Design review of the part built by this model. Coordinates are the model's own, in mm. A direction names the side the tool comes from. Coordinates: 2 decimals unless noted, no trailing zeros. Write each loop counter-clockwise with the first axis right and the second up, starting at its lowest first coordinate (ties: lowest second). Pieces come first, ordered by that corner, then holes. Notation, with made-up numbers: M 73.25,53 L 116.25,53 A10 ccw 116.25,69 Z; hole C 55.5,63 d4. An arc over 180 degrees is marked long. Return JSON: item names as keys, results as strings. Group by question number.
Autodesk Fusion 360 part; units mm, degrees
sketch "Sketch1" plane through (0, 0, 0) normal (0, 0, 1) x (1, 0, 0)
  line L0 (0, 0) -> (324.3, 0)
  line L1 (324.3, 0) -> (324.3, 429.3)
  line L2 (324.3, 429.3) -> (0, 429.3)
  line L3 (0, 429.3) -> (0, 0)
  dimension "d7" = 324.3
  dimension "d8" = 429.3
extrude "Extrude1" add sketch "Sketch1" along normal blind 55
fillet "Fillet1" radius 8 4 edges at (324.3, 0, 27.5) (324.3, 429.3, 27.5) (0, 429.3, 27.5) (0, 0, 27.5)
shell "Shell1" thickness 5 removed faces 1 at (216.2, 283.5333, 55)
ref_plane "WorkPlane1" through (162.15, 214.65, 50) normal (0, 0, 1) x (1, 0, 0)
sketch "Sketch2" plane through (0, 0, 50) normal (0, 0, 1) x (1, 0, 0)
  line L0 (10, 427.3) -> (314.3, 427.3)
  line L1 (322.3, 419.3) -> (322.3, 10)
  line L2 (314.3, 2) -> (10, 2)
  line L3 (2, 10) -> (2, 419.3)
  arc A0 (8, 424.3) -> (5, 421.3) centre (8, 421.3) ccw
  line L4 (8, 424.3) -> (316.3, 424.3)
  arc A1 (319.3, 421.3) -> (316.3, 424.3) centre (316.3, 421.3) ccw
  line L5 (319.3, 421.3) -> (319.3, 8)
  arc A2 (316.3, 5) -> (319.3, 8) centre (316.3, 8) ccw
  line L6 (316.3, 5) -> (8, 5)
  arc A3 (5, 8) -> (8, 5) centre (8, 8) ccw
  line L7 (5, 8) -> (5, 421.3)
  arc A4 (0, 8) -> (8, 0) centre (8, 8) ccw
  line L8 (8, 0) -> (316.3, 0)
  arc A5 (316.3, 0) -> (324.3, 8) centre (316.3, 8) ccw
  line L9 (324.3, 8) -> (324.3, 421.3)
  arc A6 (324.3, 421.3) -> (316.3, 429.3) centre (316.3, 421.3) ccw
  line L10 (316.3, 429.3) -> (8, 429.3)
  arc A7 (8, 429.3) -> (0, 421.3) centre (8, 421.3) ccw
  line L11 (0, 421.3) -> (0, 8)
  arc A8 (2, 10) -> (10, 2) centre (10, 10) ccw
  arc A9 (10, 427.3) -> (2, 419.3) centre (10, 419.3) ccw
  arc A10 (322.3, 419.3) -> (314.3, 427.3) centre (314.3, 419.3) ccw
  arc A11 (314.3, 2) -> (322.3, 10) centre (314.3, 10) ccw
  dimension "d19" = 2
  dimension "d20" = 2
  dimension "d21" = 2
  dimension "d22" = 2
  dimension "d23" = 8
extrude "Extrude2" cut sketch "Sketch2" along normal through all contours L0 L1 L2 L3 A8 A9 A10 A11
fillet "Fillet2" radius 8 1 faces at (216.2, 283.5333, 0)
equation "tray_depth = panel_depth + 2 * ( wall_thickness - lip_thickness ) + printer_tolerance"
equation "tray_width = panel_width + 2 * ( wall_thickness - lip_thickness ) + printer_tolerance"
equation "wall_height = 55 mm"
equation "wall_thickness = 2 mm + lip_thickness"
equation "corner_radius = 8 mm"
equation "lip_depth = 5 mm"
equation "d7 = tray_width"
equation "d8 = tray_depth"
equation "d9 = wall_height"
equation "d12 = corner_radius"
equation "d13 = wall_thickness"
equation "panel_width = 320 mm"
equation "panel_depth = 425 mm"
equation "lip_thickness = 3 mm"
equation "printer_tolerance = 0.3 mm"
equation "d19 = wall_thickness - lip_thickness"
equation "d20 = wall_thickness - lip_thickness"
equation "d21 = wall_thickness - lip_thickness"
equation "d22 = wall_thickness - lip_thickness"
equation "d23 = corner_radius"
equation "d26 = corner_radius"
Item 1: For pin 1 (2 mm diameter, centred on x = 62, y = 324, fed in from +Z), flat-tipped, find the tip position at first contact; note if it passes through.
Item 2: Add section B-B (x = 77). Write out the cut boundary in (y, z).
Item 3: Add section A-A (z = 15). Write out the cut boundary in (x, y).
Item 4: Add section C-C (y = 381). Write out the cut boundary in (x, z), plus the area to 3 significant figures.
Item 5: For line 1 (Y direction, x = 290, z = 30); line 2 (Y direction, x = 261, z = 51.5); line 3 (X direction, y = 174.5, z = 45), list the stretches that pass through material, from the lowest coordinate up.
Item 6: The part is to be moulded in two halves that separate along X. For faces 1 (the flat face through (319.3, 212, 27)), 2 (the flat face through (164, 429.3, 31)), 3 (the flat face through (0, 218, 31)), say which applies: pulls with the +X half, pulls with the -X half, needs draft (parallel to the pull), parting line crosses it, or undercut.
Item 7: Machinability: for faces 4 (the flat face through (160, 218, 0)), 5 (the flat face through (164, 424.3, 27)), which of the approach directions +Z, -Z, +X, -X, +Y, -Y give a long, thin tool a straight path to every point of the face, cutting with its end or side? Answer none if there is none.
Geometry check:
{
 "1": {"pin 1": "z = 5"},
 "2": {"outline": "M 0,8 A8 ccw 8,0 L 421.3,0 A8 ccw 429.3,8 L 429.3,55 L 427.3,55 L 427.3,50 L 424.3,50 L 424.3,5 L 5,5 L 5,50 L 2,50 L 2,55 L 0,55 Z"},
 "3": {"outline": "M 0,8 A8 ccw 8,0 L 316.3,0 A8 ccw 324.3,8 L 324.3,421.3 A8 ccw 316.3,429.3 L 8,429.3 A8 ccw 0,421.3 Z; hole M 5,8 A3 ccw 8,5 L 316.3,5 A3 ccw 319.3,8 L 319.3,421.3 A3 ccw 316.3,424.3 L 8,424.3 A3 ccw 5,421.3 Z"},
 "4": {"outline": "M 0,8 A8 ccw 8,0 L 316.3,0 A8 ccw 324.3,8 L 324.3,55 L 322.3,55 L 322.3,50 L 319.3,50 L 319.3,5 L 5,5 L 5,50 L 2,50 L 2,55 L 0,55 Z", "area": "2,060 mm^2"},
 "5": {"line 1": "0 to 5, 424.3 to 429.3", "line 2": "0 to 2, 427.3 to 429.3", "line 3": "0 to 5, 319.3 to 324.3"},
 "6": {"face 1": "undercut", "face 2": "needs draft", "face 3": "pulls with the -X half"},
 "7": {"face 4": "-Z, +X, -X, +Y, -Y", "face 5": "+Z"}
}
